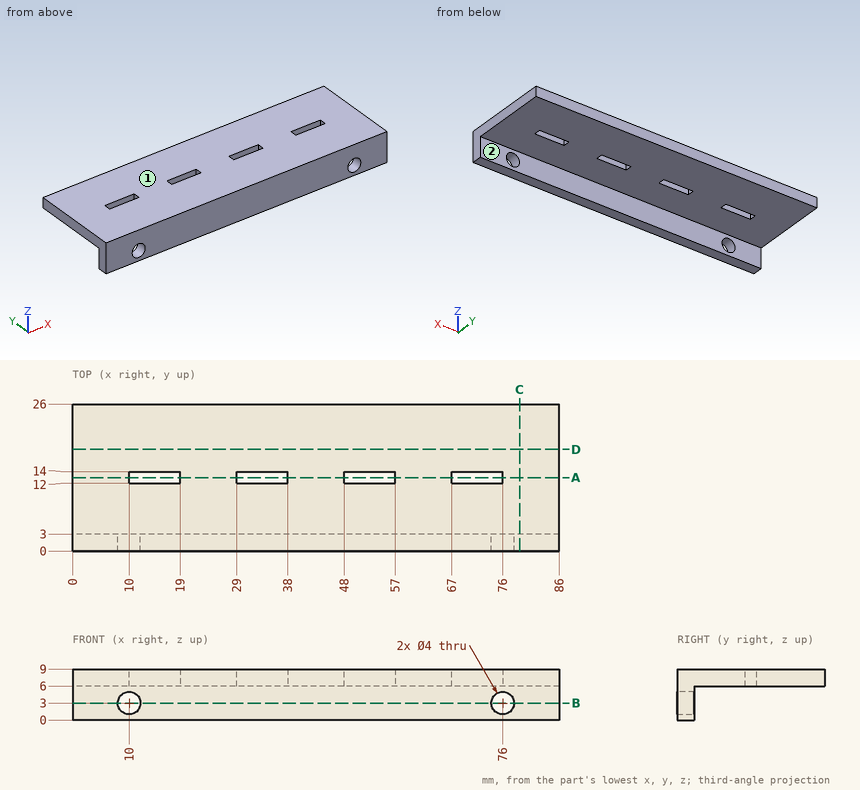
Part print with two shaded views. Sizes in mm from the minimum x, y, z corner. A direction names the side the tool comes from. Round coordinates to 2 decimals unless told otherwise and drop trailing zeros. Write each loop counter-clockwise with the first axis right and the second up, starting at its lowest first coordinate (ties: lowest second). Pieces come first, ordered by that corner, then holes. Notation, with made-up numbers: (2.25, 53.5) - (17.25, 53.5) arc R28 ccw to (17.25, 73.5) - close; hole circle Ø5 at (64, 63.5). An arc over 180 degrees is marked (long way). Answer as CSV lines item,"result".
Q1. Cut at B-B (z = 3). Write the cut outline in (x, y).
Report:
outline,"(0, 0) - (8, 0) - (8, 3) - (0, 3) - close; (12, 0) - (74, 0) - (74, 3) - (12, 3) - close; (78, 0) - (86, 0) - (86, 3) - (78, 3) - close"
Q2. Tool access for the marked faces 1 and 2: list every direction of +Z, -Z, +X, -X, +Y, -Y with a clear straight run to the whole face (end or side of a thin tool).
Report:
face 1,"+Z, +X, -X, +Y, -Y"
face 2,"-Z, +X, -X, +Y"
Q3. Cut at C-C (x = 79). Write the cut outline in (y, z).
Report:
outline,"(0, 0) - (3, 0) - (3, 6) - (26, 6) - (26, 9) - (0, 9) - close"
Q4. Drill centre lines: probe 1 along X at (y, z) = (1.6, 3); probe 2 along Z at (x, y) = (76, 0.95); probe 3 along Y at (x, z) = (36, 7.75). Where is each one in solid material? Low to high. Write a range as [from, to].
Report:
probe 1,"x = [0, 8], [12, 74], [78, 86]"
probe 2,"z = [0, 1], [5, 9]"
probe 3,"y = [0, 12], [14, 26]"
Q5. Drop flat-ended pins along their axis: pin 1 (2 mm diameter, centred on y = 12, z = 5.5, fed in from -X); pin 2 (7 mm diameter, centred on x = 38, y = 16.5, fed in from -Z); pin 3 (3.5 mm diameter, centred on x = 76, z = 3, fed in from +Y). Give the stop position or say it passes through.
Report:
pin 1,"stops at x = 0"
pin 2,"stops at z = 6"
pin 3,"passes through"
Q6. Cut at A-A (y = 13). Write the cut outline in (x, z).
Report:
outline,"(0, 6) - (10, 6) - (10, 9) - (0, 9) - close; (19, 6) - (29, 6) - (29, 9) - (19, 9) - close; (38, 6) - (48, 6) - (48, 9) - (38, 9) - close; (57, 6) - (67, 6) - (67, 9) - (57, 9) - close; (76, 6) - (86, 6) - (86, 9) - (76, 9) - close"
Q7. Cut at D-D (y = 18). Write the cut outline in (x, z).
Report:
outline,"(0, 6) - (86, 6) - (86, 9) - (0, 9) - close"
